Check sheet for the modelled part. Datum: model origin and axes. Units: mm. A direction names the side the tool comes from. Coordinates: 2 decimals unless noted, no trailing zeros. Order: outer loops, then holes, each group sorted by start corner. A loop starts at its lowest first (then second) coordinate and runs counter-clockwise, first axis right, second up.
from build123d import *

# Parameters (mm, degrees)
SKETCH1_R                                      = 38.1
BOSS_EXTRUDE1_DEPTH                            = 6.35
CBORE_FOR_4_BUTTON_HEAD_CAP_SCREW1_D           = 2.9464
CBORE_FOR_4_BUTTON_HEAD_CAP_SCREW1_CBORE_D     = 4.826
CBORE_FOR_4_BUTTON_HEAD_CAP_SCREW1_CBORE_DEPTH = 2.8448
CIRPATTERN1_COUNT                              = 8


with BuildPart() as part:
    # Sketch1 → Boss-Extrude1 (new body)
    with BuildSketch(Plane(origin=(0, 0, 0), x_dir=(1, 0, 0), z_dir=(0, 1, 0))):
        Circle(SKETCH1_R)
    extrude(amount=BOSS_EXTRUDE1_DEPTH)

    # CBORE for #4 Button Head Cap Screw1 (through all)
    with Locations(Plane(origin=(0, 0, 0), x_dir=(-1, 0, 0), z_dir=(0, -1, 0))):
        with Locations((0, -33.3375)):
            cbore_for_4_button_head_cap_screw1 = CounterBoreHole(CBORE_FOR_4_BUTTON_HEAD_CAP_SCREW1_D / 2, CBORE_FOR_4_BUTTON_HEAD_CAP_SCREW1_CBORE_D / 2, CBORE_FOR_4_BUTTON_HEAD_CAP_SCREW1_CBORE_DEPTH)

    # CirPattern1: CBORE for #4 Button Head Cap Screw1 ×8 about axis
    cirpattern1_axis = Axis((0, 0, 0), (0, 1, 0))
    for i in range(1, CIRPATTERN1_COUNT):
        add(cbore_for_4_button_head_cap_screw1.rotate(cirpattern1_axis, i * 360 / CIRPATTERN1_COUNT), mode=Mode.SUBTRACT)


solid = part.part
(1) Release check for a two-part mould opening along Z. For faces 3 (the cylindrical face through (-30.235, 3.131, 23.183)), 4 (the flat face through (-1, 6.35, -1)), 5 (the flat face through (1, 2.845, -32)) record: +Z half, -Z half, draft (parallel to the pull), parting line (faces both ways), or undercut.
Filled in:
face 3: parting line
face 4: draft
face 5: undercut
(2) Tool access check on faces 1 (the flat face through (-24, 2.845, 22)), 2 (the cylindrical face through (22.4, 4.62, 22.68)). Record the directions out of +Z, -Z, +X, -X, +Y, -Y that give a thin tool (end or side, any length) a straight path to the whole face; none if there is none.
Filled in:
face 1: -Y
face 2: +Y, -Y
(3) Cross-section at C-C (y = 4.25). Count the separate pieces of the cut face and the enclosed holes in it, and give its area (3 significant figures).
Filled in:
separate pieces: 1
enclosed holes: 8
area: 4,510 mm2
(4) Cross-section at B-B (x = 0). Enter the section's corners in (y, z), and give its area (3 significant figures).
Filled in:
outline: (0, -38.1) - (6.35, -38.1) - (6.35, -34.81) - (2.84, -34.81) - (2.84, -35.75) - (0, -35.75) - close; (0, -30.92) - (2.84, -30.92) - (2.84, -31.86) - (6.35, -31.86) - (6.35, 31.86) - (2.84, 31.86) - (2.84, 30.92) - (0, 30.92) - close; (0, 35.75) - (2.84, 35.75) - (2.84, 34.81) - (6.35, 34.81) - (6.35, 38.1) - (0, 38.1) - close
area: 436 mm2
(5) Thickness scan on probe 1 along Z at (x, y) = (0, 1.05); probe 2 along Z at (x, y) = (0, 5.65). Record the ranges inside material, lowest first.
Filled in:
probe 1: z = -38.1 to -35.75, -30.92 to 30.92, 35.75 to 38.1
probe 2: z = -38.1 to -34.81, -31.86 to 31.86, 34.81 to 38.1
(6) Cross-section at A-A (z = 0). Enter the section's corners in (x, y).
Filled in:
outline: (-38.1, 0) - (-35.75, 0) - (-35.75, 2.84) - (-34.81, 2.84) - (-34.81, 6.35) - (-38.1, 6.35) - close; (-31.86, 2.84) - (-30.92, 2.84) - (-30.92, 0) - (30.92, 0) - (30.92, 2.84) - (31.86, 2.84) - (31.86, 6.35) - (-31.86, 6.35) - close; (34.81, 2.84) - (35.75, 2.84) - (35.75, 0) - (38.1, 0) - (38.1, 6.35) - (34.81, 6.35) - close
(7) Go/stop test with flat-tipped pins: P1, Ø1.5, axis at y = 1.5, z = -24, coming from the -X side; P2, Ø2.5, axis at x = 24.5, z = 24, coming from the -Y side; P3, Ø3, axis at y = 5, z = 3.5, coming from the -X side. Record where each tip stops, or that it passes through.
Filled in:
P1: stops at x = -30.18
P2: stops at y = 2.84
P3: stops at x = -38.05
(8) Cross-section at D-D (x = 27.5). Enter the section's corners in (y, z), and give its area (3 significant figures).
Filled in:
outline: (0, -26.37) - (6.35, -26.37) - (6.35, 26.37) - (0, 26.37) - close
area: 335 mm2
